from build123d import *

# Parameters (mm, degrees)
PAD_DEPTH                = 30
PAD_DEPTH_BACK           = 30
SKETCH001_R              = 11.05
SKETCH001_R_2            = 1.5
POCKET_DEPTH             = 5.54
SKETCH002_R              = 1.5
POCKET001_DEPTH          = 20.001
CLONE001_PITCH_ANGLE     = 90
CLONE001_PLACEMENT_ANGLE = -90


with BuildPart() as part:
    # Sketch → Pad (new body, two sides)
    with BuildSketch(Plane.XZ) as pad_sk:
        Polygon((-10, -20), (-10, 0), (10, 0), (10, -2), (-8, -2), (-8, -20), align=None)
    extrude(amount=PAD_DEPTH)
    extrude(pad_sk.sketch, amount=-PAD_DEPTH_BACK)

    # Sketch001 (on Face4 of Pad) → Pocket (cut)
    with BuildSketch(Plane(origin=(13, 0, -2), x_dir=(1, 0, 0), z_dir=(0, 0, -1))):
        Circle(SKETCH001_R)
        with Locations((-15.5, 15.5)):
            Circle(SKETCH001_R_2)
        with Locations((15.5, 15.5)):
            Circle(SKETCH001_R_2)
        with Locations((15.5, -15.5)):
            Circle(SKETCH001_R_2)
        with Locations((-15.5, -15.5)):
            Circle(SKETCH001_R_2)
    extrude(amount=-POCKET_DEPTH, mode=Mode.SUBTRACT)

    # Sketch002 (on Face1 of Pocket) → Pocket001 (cut, through all)
    with BuildSketch(Plane(origin=(-10, 0, 0), x_dir=(0, 0, -1), z_dir=(-1, 0, 0))):
        with Locations((10, 26)):
            Circle(SKETCH002_R)
        with Locations((10, -26)):
            Circle(SKETCH002_R)
    extrude(amount=-POCKET001_DEPTH, mode=Mode.SUBTRACT)


with BuildPart() as part_1:
    # Clone001 pitch: moved
    add(part.part.rotate(Axis((0, 0, 0), (0, 1, 0)), CLONE001_PITCH_ANGLE))


with BuildPart() as part_2:
    # Clone001 placement: moved
    add(part_1.part.moved(Location((0, 0, -10))).rotate(Axis((0, 0, -10), (0, 0, 1)), CLONE001_PLACEMENT_ANGLE))


solid = part_2.part
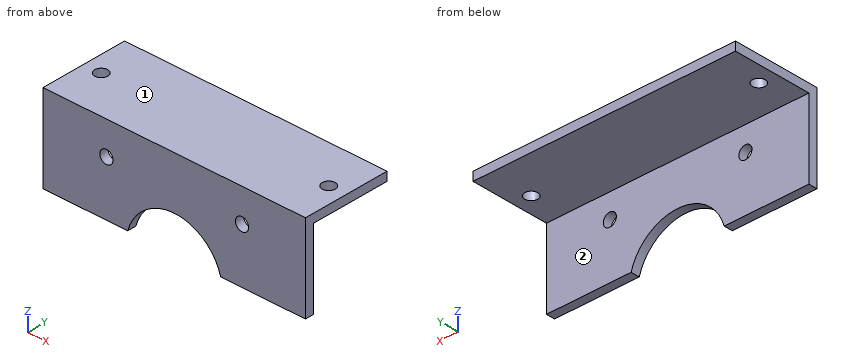
The listing builds one solid part. Answer for the finished solid, in the listing's coordinates (mm). Face numbers are marked on the shaded views. A direction names the side the tool comes from. Give positions to 0.01 mm unless a question says otherwise; leave off trailing zeros. Write each loop counter-clockwise with the first axis right and the second up, starting at its lowest first coordinate (ties: lowest second). Pieces come first, ordered by that corner, then holes. Notation, with made-up numbers: (-17.5, -21.5) - (10.5, -21.5) arc R26 ccw to (10.5, 16.5) - close; hole circle Ø11 at (-14, -39.75). An arc over 180 degrees is marked (long way). One line per question, with ' | ' between items. Start each with the question number.
1. Section B-B, the plane z = -16 is taken. Determine the outline of the cut face in (x, y), then the cut area to 3 significant figures.
2. Section C-C, the plane x = 26 is taken. Determine the outline of the cut face in (y, z), then the cut area to 3 significant figures.
3. Given P1, Ø6, axis at x = 14, z = -11.5, coming from the +Y side; P2, Ø10, axis at y = 2.5, z = -15, coming from the -X side, each flat-ended and moving along its own axis, determine where each tip first touches the part or whether it passes through.
4. Straight lines are drawn through the part: line 1 (X direction, y = 0.4, z = -7.5); line 2 (X direction, y = 10, z = -0.4); line 3 (Z direction, x = 15.5, y = 1.3). For each, find the intervals that lie inside material, in ascending order.
5. Section A-A, the plane y = 10 is taken. Determine the outline of the cut face in (x, z), then the cut area to 3 significant figures.
6. Section D-D, the plane z = -7.5 is taken. Determine the outline of the cut face in (x, y).
7. For the marked faces 1 and 2, determine the directions among +Z, -Z, +X, -X, +Y, -Y from which every point of the face is accessible in a straight line to the end or side of a thin tool.
Result:
1) outline: (-30, 0) - (-8.55, 0) - (-8.55, 2) - (-30, 2) - close; (8.55, 0) - (30, 0) - (30, 2) - (8.55, 2) - close | area: 85.8 mm2
2) outline: (0, -20) - (2, -20) - (2, -2) - (8.5, -2) - (8.5, 0) - (0, 0) - close; (11.5, -2) - (20, -2) - (20, 0) - (11.5, 0) - close | area: 70.0 mm2
3) P1: stops at y = 2 | P2: stops at x = -30
4) line 1: x = -30 to -17, -14 to 14, 17 to 30 | line 2: x = -30 to -27.5, -24.5 to 24.5, 27.5 to 30 | line 3: z = -20 to -9, -6 to 0
5) outline: (-30, -2) - (-27.5, -2) - (-27.5, 0) - (-30, 0) - close; (-24.5, -2) - (24.5, -2) - (24.5, 0) - (-24.5, 0) - close; (27.5, -2) - (30, -2) - (30, 0) - (27.5, 0) - close | area: 108 mm2
6) outline: (-30, 0) - (-17, 0) - (-17, 2) - (-30, 2) - close; (-14, 0) - (14, 0) - (14, 2) - (-14, 2) - close; (17, 0) - (30, 0) - (30, 2) - (17, 2) - close
7) face 1: +Z, +X, -X, +Y, -Y | face 2: -Z, +X, -X, +Y
